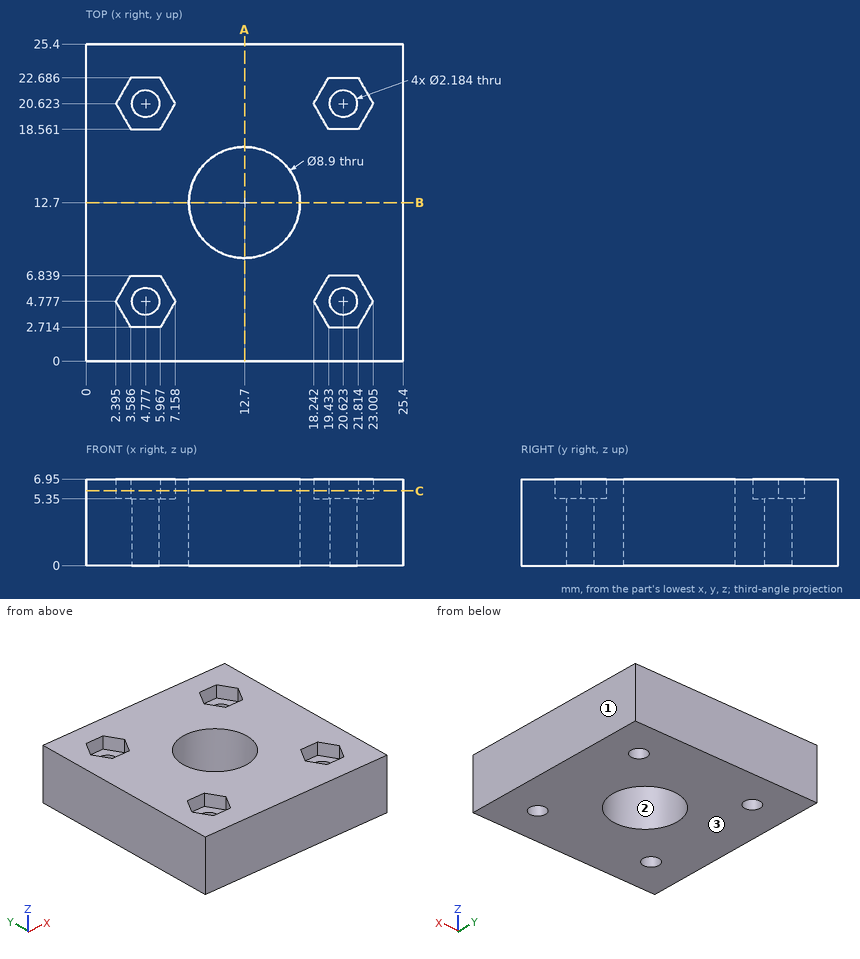
Here's the drawing with two shaded views (mm, measured from the low corner). I have some questions. Round coordinates to 2 decimals unless told otherwise and drop trailing zeros. Write each loop counter-clockwise with the first axis right and the second up, starting at its lowest first coordinate (ties: lowest second). Pieces come first, ordered by that corner, then holes.
(1) Suppose I cut it at C-C on z = 6. State how many separate pieces and enclosed holes the cut face has, and give its area (3 significant figures).
Findings below:
separate pieces: 1
enclosed holes: 5
area: 524 mm2
(2) Suppose I cut it at A-A on x = 12.7. Write out the boundary of the cut face in (y, z), and give its area (3 significant figures).
Findings below:
outline: (0, 0) - (8.25, 0) - (8.25, 6.95) - (0, 6.95) - close; (17.15, 0) - (25.4, 0) - (25.4, 6.95) - (17.15, 6.95) - close
area: 115 mm2
(3) If I drill on probe 1 along X at (y, z) = (20.75, 1.5); probe 2 along Y at (x, z) = (5.25, 2.5); probe 3 along Y at (x, z) = (12.7, 3.75), over which ranges is the centre line in solid material (lowest first)?
Findings below:
probe 1: x = 0 to 3.69, 5.86 to 19.54, 21.71 to 25.4
probe 2: y = 0 to 3.79, 5.76 to 19.64, 21.61 to 25.4
probe 3: y = 0 to 8.25, 17.15 to 25.4
(4) Thinking about a two-plate mould opening in X: for the marked faces 1, 2 and 3, which applies, +X half, -X half, draft (parallel to the pull), parting line (faces both ways), or undercut?
Findings below:
face 1: +X half
face 2: undercut
face 3: draft
(5) For pin 1 (3.5 mm diameter, centred on x = 21, y = 6, fed in from +Z); pin 2 (2 mm diameter, centred on x = 4.5, y = 21.5, fed in from +Z), each with a flat end and sliding along its axis, tell me the tip position at first contact or that it passes through.
Findings below:
pin 1: stops at z = 6.95
pin 2: stops at z = 5.35
